Geometry: final body of the model. Coordinates: model frame, mm. A direction names the side the tool comes from. Round coordinates to 2 decimals unless told otherwise and drop trailing zeros. Loops run counter-clockwise (first coordinate to the right, second up) from the corner with the lowest first, then second, coordinate; pieces in that order, holes last. Notation, with made-up numbers: M 68,-25.75 L 120,-25.75 A6 cw 120,-18.75 Z; hole C 47,-18.5 d1. An arc over 180 degrees is marked long. Answer as a JSON object with one key per item and string values.
```python
from build123d import *

# Parameters (mm, degrees)
EXTRUDE_309_DEPTH      = 1.2
SKETCH_2_W             = 32
SKETCH_2_H             = 1.2
PCB_DEPTH              = 6.5
PCB_2_DEPTH            = 6
CUT_EXTRUDE_1014_REACH = 54.571
SKETCH_5_W             = 32
SKETCH_5_H             = 1.2
EXTRUDE_1286_DEPTH     = 4


with BuildPart() as part:
    # 草图1 → Extrude 309 (new body)
    with BuildSketch(Plane(origin=(0, 0, 0), x_dir=(1, 0, 0), z_dir=(0, 1, 0))):
        Polygon((32, 0), (32, 40), (32, 41.2), (0, 41.2), (0, 40), (0, 0), (0, -1.2), (32, -1.2), align=None)
    extrude(amount=EXTRUDE_309_DEPTH)

    # 草图2 → PCB (add)
    with BuildSketch(Plane(origin=(0, 1.2, 0), x_dir=(1, 0, 0), z_dir=(0, 1, 0))):
        with Locations((16, -0.6)):
            Rectangle(SKETCH_2_W, SKETCH_2_H)
        with Locations((16, 40.6)):
            Rectangle(SKETCH_2_W, SKETCH_2_H)
    extrude(amount=PCB_DEPTH)

    # 草图3 → PCB 2 (add)
    with BuildSketch(Plane(origin=(0, 1.2, 0), x_dir=(1, 0, 0), z_dir=(0, 1, 0))):
        Polygon((16, 0), (25.6, 0), (25.6, 1.5), (6.4, 1.5), (6.4, 0), align=None)
    extrude(amount=PCB_2_DEPTH)

    # 草图4 → Cut-Extrude 1014 (cut, up to next)
    with BuildSketch(Plane(origin=(0, 1.2, 0), x_dir=(1, 0, 0), z_dir=(0, 1, 0)), mode=Mode.PRIVATE) as cut_extrude_1014_sk1:
        Polygon((16, 40), (26, 40), (26, 32), (6, 32), (6, 40), align=None)
    cut_extrude_1014_tool1 = extrude(cut_extrude_1014_sk1.sketch, amount=-CUT_EXTRUDE_1014_REACH, mode=Mode.PRIVATE) & part.part
    add(cut_extrude_1014_tool1.solids().sort_by_distance((16, 1.2, -36))[0], mode=Mode.SUBTRACT)

    # 草图5 → Extrude 1286 (add)
    with BuildSketch(Plane.XZ):
        with Locations((16, 0.6)):
            Rectangle(SKETCH_5_W, SKETCH_5_H)
        with Locations((16, -40.6)):
            Rectangle(SKETCH_5_W, SKETCH_5_H)
    extrude(amount=EXTRUDE_1286_DEPTH)


solid = part.part
```
1) Cut plane D-D on y = 0.5. Return the cut outline in (x, z).
Geometry results:
{"outline": "M 0,-41.2 L 32,-41.2 L 32,1.2 L 0,1.2 Z; hole M 6,-40 L 26,-40 L 26,-32 L 6,-32 Z"}
2) Cut plane A-A on x = 7. Return the cut outline in (y, z).
Geometry results:
{"outline": "M -4,-41.2 L 7.7,-41.2 L 7.7,-40 L -4,-40 Z; M -4,0 L 0,0 L 0,-32 L 1.2,-32 L 1.2,-1.5 L 7.2,-1.5 L 7.2,0 L 7.7,0 L 7.7,1.2 L -4,1.2 Z"}
3) Cut plane B-B on y = -3. Return the cut outline in (x, z).
Geometry results:
{"outline": "M 0,-41.2 L 32,-41.2 L 32,-40 L 0,-40 Z; M 0,0 L 32,0 L 32,1.2 L 0,1.2 Z"}
4) Set-up query: faces 1 (the face through (26, 1, -36)), 2 (the face through (16, 0, -20)), 3 (the face through (26, 4, 0)), 4 (the face through (16, 7.2, -1)), 5 (the face through (6.4, 4, -1)). Return all of +Z, -Z, +X, -X, +Y, -Y with unobstructed straight access to the full face (end or side cutting, diameter ignored); none if empty.
Geometry results:
{"face 1": "+Y, -Y", "face 2": "+X, -X, -Y", "face 3": "+Y", "face 4": "+X, -X, +Y", "face 5": "-X, +Y"}
5) Pull-direction query (Z, two-part tool) for faces 6 (the face through (16, 2, -41.2)), 7 (the face through (16, 2, 1.2)), 8 (the face through (32, 1, -20)), 9 (the face through (25.6, 4, -1)); classes: +Z half, -Z half, draft (parallel to the pull), parting line (faces both ways), or undercut.
Geometry results:
{"face 6": "-Z half", "face 7": "+Z half", "face 8": "draft", "face 9": "undercut"}
6) First-contact query: pin 1 (8 mm diameter, centred on x = 24.5, z = -7.5, fed in from -Y); pin 2 (0.8 mm diameter, centred on y = 4, z = -1, fed in from -X); pin 3 (9.5 mm diameter, centred on x = 10, z = -26.5, fed in from +Y); pin 4 (6 mm diameter, centred on y = 0, z = -7, fed in from -X). Flat tips, straight axial feed; report the tip coordinate or a pass-through.
Geometry results:
{"pin 1": "y = 0", "pin 2": "x = 6.4", "pin 3": "y = 1.2", "pin 4": "x = 0"}
7) Cut plane C-C on z = -38. Return the cut outline in (x, y), and give its area (3 significant figures).
Geometry results:
{"outline": "M 0,0 L 6,0 L 6,1.2 L 0,1.2 Z; M 26,0 L 32,0 L 32,1.2 L 26,1.2 Z", "area": "14.4 mm2"}
8) Line query: probe 1 along Z at (x, y) = (31, -0.75); probe 2 along Z at (x, y) = (13.5, 1); probe 3 along Y at (x, z) = (6.5, -1). Output: solid intervals per line, ascending.
Geometry results:
{"probe 1": "-41.2 to -40, 0 to 1.2", "probe 2": "-41.2 to -40, -32 to 1.2", "probe 3": "0 to 7.2"}
